```python
from build123d import *

# Parameters (mm, degrees)
F0_W     = 22.225
F0_H     = 50.2666
F1_DEPTH = 6.6294
F2_W     = 17.3609
F2_H     = 7.4041
F3_DEPTH = 1.9558
F4_W     = 0.635
F4_H     = 0.635
F5_DEPTH = 5.715
F6_SIZE  = 0.1778


with BuildPart() as f1:
    # F0 (on Top) → F1 (new body)
    with BuildSketch(Plane.XY):
        Rectangle(F0_W, F0_H)
    extrude(amount=F1_DEPTH)

    # F2 (on face) → F3 (join)
    with BuildSketch(Plane.XY.offset(6.6294)):
        with Locations((0, 20.08505)):
            Rectangle(F2_W, F2_H)
    extrude(amount=F3_DEPTH)

    # F4 (on face) → F5 (join)
    with BuildSketch(Plane.XY.offset(8.5852)):
        with Locations((7.51205, 22.6441)):
            Rectangle(F4_W, F4_H)
        with Locations((5.09905, 22.6441)):
            Rectangle(F4_W, F4_H)
        with Locations((2.68605, 22.6441)):
            Rectangle(F4_W, F4_H)
        with Locations((0.27305, 22.6441)):
            Rectangle(F4_W, F4_H)
        with Locations((-2.13995, 22.6441)):
            Rectangle(F4_W, F4_H)
        with Locations((-4.55295, 22.6441)):
            Rectangle(F4_W, F4_H)
        with Locations((-6.96595, 22.6441)):
            Rectangle(F4_W, F4_H)
        with Locations((-6.96595, 20.1041)):
            Rectangle(F4_W, F4_H)
        with Locations((-4.55295, 20.1041)):
            Rectangle(F4_W, F4_H)
        with Locations((-2.13995, 20.1041)):
            Rectangle(F4_W, F4_H)
        with Locations((0.27305, 20.1041)):
            Rectangle(F4_W, F4_H)
        with Locations((2.68605, 20.1041)):
            Rectangle(F4_W, F4_H)
        with Locations((5.09905, 20.1041)):
            Rectangle(F4_W, F4_H)
        with Locations((7.51205, 20.1041)):
            Rectangle(F4_W, F4_H)
        with Locations((-6.96595, 17.5641)):
            Rectangle(F4_W, F4_H)
        with Locations((-4.55295, 17.5641)):
            Rectangle(F4_W, F4_H)
        with Locations((-2.13995, 17.5641)):
            Rectangle(F4_W, F4_H)
        with Locations((0.27305, 17.5641)):
            Rectangle(F4_W, F4_H)
        with Locations((2.68605, 17.5641)):
            Rectangle(F4_W, F4_H)
        with Locations((5.09905, 17.5641)):
            Rectangle(F4_W, F4_H)
        with Locations((7.51205, 17.5641)):
            Rectangle(F4_W, F4_H)
    extrude(amount=F5_DEPTH)

    # F6
    f6_edges = [f1.edges().sort_by_distance(p)[0] for p in [
        (-6.96595, 22.9616, 14.3002),
        (-7.28345, 22.6441, 14.3002),
        (-6.96595, 22.3266, 14.3002),
        (-6.64845, 22.6441, 14.3002),
        (-6.64845, 20.1041, 14.3002),
        (-6.96595, 20.4216, 14.3002),
        (-7.28345, 20.1041, 14.3002),
        (-6.96595, 19.7866, 14.3002),
        (-4.55295, 22.9616, 14.3002),
        (-4.87045, 22.6441, 14.3002),
        (-4.55295, 22.3266, 14.3002),
        (-4.23545, 22.6441, 14.3002),
        (-4.55295, 20.4216, 14.3002),
        (-4.87045, 20.1041, 14.3002),
        (-4.55295, 19.7866, 14.3002),
        (-4.23545, 20.1041, 14.3002),
        (-6.64845, 17.5641, 14.3002),
        (-6.96595, 17.8816, 14.3002),
        (-7.28345, 17.5641, 14.3002),
        (-6.96595, 17.2466, 14.3002),
        (-4.55295, 17.8816, 14.3002),
        (-4.87045, 17.5641, 14.3002),
        (-4.55295, 17.2466, 14.3002),
        (-4.23545, 17.5641, 14.3002),
        (-2.13995, 20.4216, 14.3002),
        (-2.45745, 20.1041, 14.3002),
        (-2.13995, 19.7866, 14.3002),
        (-1.82245, 20.1041, 14.3002),
        (-2.13995, 22.9616, 14.3002),
        (-2.45745, 22.6441, 14.3002),
        (-2.13995, 22.3266, 14.3002),
        (-1.82245, 22.6441, 14.3002),
        (-2.13995, 17.8816, 14.3002),
        (-2.45745, 17.5641, 14.3002),
        (-2.13995, 17.2466, 14.3002),
        (-1.82245, 17.5641, 14.3002),
        (0.27305, 17.8816, 14.3002),
        (-0.04445, 17.5641, 14.3002),
        (0.27305, 17.2466, 14.3002),
        (0.59055, 17.5641, 14.3002),
        (0.27305, 20.4216, 14.3002),
        (-0.04445, 20.1041, 14.3002),
        (0.27305, 19.7866, 14.3002),
        (0.59055, 20.1041, 14.3002),
        (0.27305, 22.9616, 14.3002),
        (-0.04445, 22.6441, 14.3002),
        (0.27305, 22.3266, 14.3002),
        (0.59055, 22.6441, 14.3002),
        (2.68605, 22.9616, 14.3002),
        (2.36855, 22.6441, 14.3002),
        (2.68605, 22.3266, 14.3002),
        (3.00355, 22.6441, 14.3002),
        (2.36855, 20.1041, 14.3002),
        (2.68605, 19.7866, 14.3002),
        (2.68605, 20.4216, 14.3002),
        (3.00355, 20.1041, 14.3002),
        (2.68605, 17.8816, 14.3002),
        (2.36855, 17.5641, 14.3002),
        (2.68605, 17.2466, 14.3002),
        (3.00355, 17.5641, 14.3002),
        (5.09905, 20.4216, 14.3002),
        (4.78155, 20.1041, 14.3002),
        (5.09905, 19.7866, 14.3002),
        (5.41655, 20.1041, 14.3002),
        (5.09905, 17.8816, 14.3002),
        (4.78155, 17.5641, 14.3002),
        (5.09905, 17.2466, 14.3002),
        (5.41655, 17.5641, 14.3002),
        (5.09905, 22.9616, 14.3002),
        (4.78155, 22.6441, 14.3002),
        (5.09905, 22.3266, 14.3002),
        (5.41655, 22.6441, 14.3002),
        (7.19455, 20.1041, 14.3002),
        (7.51205, 19.7866, 14.3002),
        (7.82955, 20.1041, 14.3002),
        (7.51205, 20.4216, 14.3002),
        (7.19455, 17.5641, 14.3002),
        (7.51205, 17.2466, 14.3002),
        (7.82955, 17.5641, 14.3002),
        (7.51205, 17.8816, 14.3002),
        (7.51205, 22.9616, 14.3002),
        (7.19455, 22.6441, 14.3002),
        (7.51205, 22.3266, 14.3002),
        (7.82955, 22.6441, 14.3002),
    ]]
    chamfer(f6_edges, length=F6_SIZE)


solid = f1.part
```
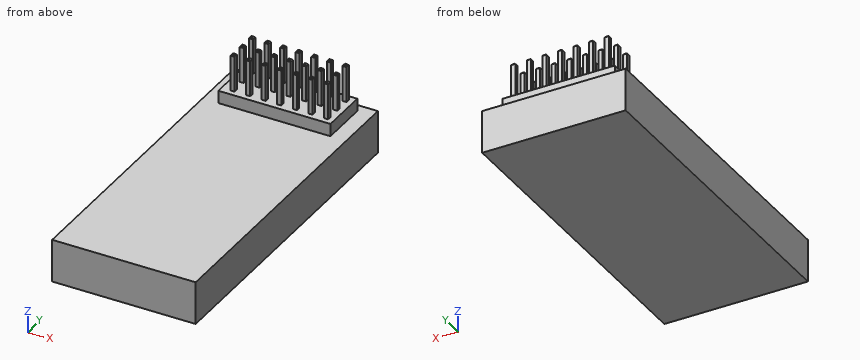
Model file for the job. Use its own axes, mm. Give positions to 0.01 mm unless a question says otherwise; leave off trailing zeros. Write each loop counter-clockwise with the first axis right and the second up, starting at its lowest first coordinate (ties: lowest second). Pieces come first, ordered by that corner, then holes. Notation, with made-up numbers: (2, 18.5) - (19, 18.5) arc R12 ccw to (19, 24.5) - close; hole circle Ø7 at (-13.5, 17). An arc over 180 degrees is marked (long way). One line per question, with ' | ' between items. Start each with the question number.
(1) Slice it at C-C on x = -9.5. Write the cut outline in (y, z).
(2) Pin check, flat tips, straight feed: P1, Ø6, axis at x = 2.5, z = 12, coming from the +Y side; P2, Ø0.5, axis at x = -7, z = 11.5, coming from the -Y side; P3, Ø3, axis at x = -1.5, y = 13, coming from the +Z side. Stop position of each tip, or through.
(3) Slice it at D-D on z = 7.75. Write the cut outline in (x, y).
(4) Slice it at A-A on y = 21. Write the cut outline in (x, z), plus the area to 3 significant figures.
(5) Slice it at B-B on z = 11.25. Give the number of separate pieces and of enclosed holes in the cut face, plus the area to 3 significant figures.
(6) Wall check: line 1 along Y through (x, z) = (7.75, 11.25); line 2 along Y through (x, z) = (0, 7.75); line 3 along Z through (x, y) = (4.25, -22). Give the ranges that are in metal, low to high. Write a range as from..to.
Results below:
1) outline: (-25.13, 0) - (25.13, 0) - (25.13, 6.63) - (-25.13, 6.63) - close
2) P1: y = 22.96 | P2: y = 17.25 | P3: z = 6.63
3) outline: (-8.68, 16.38) - (8.68, 16.38) - (8.68, 23.79) - (-8.68, 23.79) - close
4) outline: (-11.11, 0) - (11.11, 0) - (11.11, 6.63) - (8.68, 6.63) - (8.68, 8.59) - (-8.68, 8.59) - (-8.68, 6.63) - (-11.11, 6.63) - close | area: 181 mm^2
5) separate pieces: 21 | enclosed holes: 0 | area: 8.47 mm^2
6) line 1: 17.25..17.88, 19.79..20.42, 22.33..22.96 | line 2: 16.38..23.79 | line 3: 0..6.63
